```python
from build123d import *

# Parameters (mm, degrees)
F0_R     = 6
F1_DEPTH = 25
F2_W     = 18
F2_H     = 9
F3_DEPTH = 12.5
F4_R     = 10


with BuildPart() as f1:
    # F0 (on Front) → F1 (new body)
    with BuildSketch(Plane.XZ):
        with BuildLine():
            Line((77, 6), (10.965856, 6))
            ThreePointArc((10.965856, 6), (-12.5, 0), (10.965856, -6))
            Line((10.965856, -6), (77, -6))
            ThreePointArc((77, -6), (95, 0), (77, 6))
        make_face()
        Circle(F0_R, mode=Mode.SUBTRACT)
        with Locations((85, 0)):
            Circle(F0_R, mode=Mode.SUBTRACT)
    extrude(amount=F1_DEPTH)

    # F2 (on Top) → F3 (intersect, symmetric)
    with BuildSketch(Plane.XY):
        Polygon((20, 0), (-12.5, 0), (-12.5, -9), (19.212602, -9), (64.582857, -17), (77, -17), (77, -8), (65.370255, -8), align=None)
        with Locations((86, -12.5)):
            Rectangle(F2_W, F2_H)
    extrude(amount=F3_DEPTH, both=True, mode=Mode.INTERSECT)

    # F4
    f4_edges = [f1.edges().sort_by_distance(p)[0] for p in [
        (10.965856, -4.5, 6),
        (77, -12.5, 6),
        (20, 0, 0),
        (65.370255, -8, 0),
        (77, -12.5, -6),
        (10.965856, -4.5, -6),
        (64.582857, -17, 0),
        (19.212602, -9, 0),
    ]]
    fillet(f4_edges, radius=F4_R)


solid = f1.part
```
Here's how the part is built. I have some questions about the finished solid (model axes, mm). A direction names the side the tool comes from. Round coordinates to 2 decimals unless told otherwise and drop trailing zeros. Write each loop counter-clockwise with the first axis right and the second up, starting at its lowest first coordinate (ties: lowest second). Pieces come first, ordered by that corner, then holes.
Q1. If we section it at D-D on x = 0: Write out the boundary of the cut face in (y, z), plus the area to 3 significant figures.
Q2. If we section it at C-C on y = -13: Write out the boundary of the cut face in (x, z), plus the area to 3 significant figures.
Q3. Will these pins go through, and if not, where does the flat tip stop? P1, Ø10, axis at y = -7, z = 9.5, coming from the -X side; P2, Ø8.5, axis at x = 58, y = -12, coming from the -Z side; P3, Ø6, axis at x = 83, y = -14.5, coming from the +Z side.
Q4. Which directions (+Z, -Z, +X, -X, +Y, -Y) give clear straight access to the entire face, cutting with the end or side of a thin tool? Please do faces 4 (the flat face through (6, -9, -3)), 5 (the flat face through (45, -8, 6)), 6 (the flat face through (78, -8, 0)).
Q5. If we mould it in two halves opening along Z, with no side actions, what happens to faces 1 (the cylindrical face through (64.598, -16.963, 0.084)), 2 (the cylindrical face through (-6, -4, 0)), 3 (the cylindrical face through (12.07, -4.56, 6.73))? For each: +Z half, -Z half, draft (parallel to the pull), parting line (faces both ways), or undercut.
Q6. If we section it at A-A on x = 85: Write out the boundary of the cut face in (y, z).
Q7. If we section it at B-B on z = 3: Write out the boundary of the cut face in (x, y), plus the area to 3 significant figures.
Q8. Please list where these lines run through material, in increasing order: probe 1 along Z at (x, y) = (85, -13); probe 2 along Y at (x, z) = (80, 5); probe 3 along Y at (x, z) = (-5, 8.5).
Answer below:
1. outline: (-9, -12.5) - (0, -12.5) - (0, -6) - (-9, -6) - close; (-9, 6) - (0, 6) - (0, 12.5) - (-9, 12.5) - close
1. area: 117 mm2
2. outline: (41.9, -6) - (73, -6) arc R10 cw to (79, -8) arc R10 ccw (long way) to (79, 8) arc R10 cw to (73, 6) - (41.9, 6) - close; hole circle Ø12 at (85, 0)
2. area: 609 mm2
3. P1: stops at x = -11.66
3. P2: stops at z = -6
3. P3: stops at z = 10
4. face 4: +Z, -Z, -X, -Y
4. face 5: +Z, +Y, -Y
4. face 6: +Z, -Z, +X, +Y
5. face 1: draft
5. face 2: undercut
5. face 3: +Z half
6. outline: (-17, -10) - (-8, -10) - (-8, -6) - (-17, -6) - close; (-17, 6) - (-8, 6) - (-8, 10) - (-17, 10) - close
7. outline: (-12.13, -9) - (-5.2, -9) - (-5.2, 0) - (-12.13, 0) - close; (5.2, -9) - (18.34, -9) arc R10 cw to (20.07, -9.15) - (63.72, -16.85) arc R10 ccw to (65.46, -17) - (79.8, -17) - (79.8, -8) - (66.25, -8) arc R10 cw to (64.51, -7.85) - (20.86, -0.15) arc R10 ccw to (19.13, 0) - (5.2, 0) - close; (90.2, -17) - (94.54, -17) - (94.54, -8) - (90.2, -8) - close
7. area: 779 mm2
8. probe 1: z = -10 to -6, 6 to 10
8. probe 2: y = -17 to -8
8. probe 3: y = -9 to 0
